Read the model definition and answer for the solid it produces. Units are mm, in the model's axes. A direction names the side the tool comes from. Round coordinates to 2 decimals unless told otherwise and drop trailing zeros. Write each loop counter-clockwise with the first axis right and the second up, starting at its lowest first coordinate (ties: lowest second). Pieces come first, ordered by that corner, then holes. Notation, with made-up numbers: (-33.75, 2) - (4.25, 2) arc R13 ccw to (4.25, 26) - close; hole circle Ø3 at (68.25, -30). An arc over 180 degrees is marked (long way). One line per item, written item: value. Start each with the question number.
(1) For faces 1 (the face through (36.164, 61.944, -12.114)), 2 (the face through (-30, 62, -5.797)), determine the directions among +Z, -Z, +X, -X, +Y, -Y from which every point of the face is accessible in a straight line to the end or side of a thin tool.
(2) A cutting plane is placed at B-B, the plane y = 21.5. Determine the outline of the cut face in (x, z), plus the area to 3 significant figures.
(3) A cutting plane is placed at C-C, the plane x = -8.5. Determine the outline of the cut face in (y, z).
(4) Find the intervals of material crossed by L1, parallel to Y at x = -16.5, z = -3.75; L2, parallel to X at y = 44.5, z = -0.5; L3, parallel to Z at x = -8.5, y = 5, in increasing order.
(5) The mould has two halves that part along Y. Classify faces 3 (the face through (-1.464, 4.056, -1.122)), 4 (the face through (15, 58, -6)), 5 (the face through (-13, 66, -4)): +Y half, -Y half, draft (parallel to the pull), parting line (faces both ways), or undercut.
(6) Flat-ended cylindrical pins translate along their axes: pin 1 Ø8 at (x, y) = (-16, 52.5) entering from +Z; pin 2 Ø2 at (y, z) = (53, -5) entering from -X; pin 3 Ø1.8 at (x, z) = (-35.79, -0.8) entering from +Y (1 decimal); pin 4 Ø2.5 at (x, y) = (-30, 63) entering from -Z. Find the tip coordinate at first contact, or state that the pin passes through.
(7) A cutting plane is placed at A-A, the plane x = -53. Determine the outline of the cut face in (y, z), plus the area to 3 significant figures.
from build123d import *

# Parameters (mm, degrees)
BOSS_EXTRUDE1_DEPTH = 8
SKETCH2_R           = 1.7
SKETCH2_R_2         = 1.5
CUT_EXTRUDE1_DEPTH  = 10
FILLET1_SIZE        = 5
SKETCH3_R           = 5
BOSS_EXTRUDE2_DEPTH = 25


with BuildPart() as part:
    # Sketch1 → Boss-Extrude1 (new body)
    with BuildSketch(Plane(origin=(0, 0, 0), x_dir=(1, 0, 0), z_dir=(0, 1, 0))):
        Polygon((0, 5.796570021), (-65, 5.796570021), (-65, -4.203429979), (0, -4.203429979), (42, 8.002969552), (39.5, 17.276398151), align=None)
    extrude(amount=BOSS_EXTRUDE1_DEPTH)

    # Sketch2 → Cut-Extrude1 (cut)
    with BuildSketch(Plane(origin=(0, 8, 0), x_dir=(1, 0, 0), z_dir=(0, 1, 0))):
        with Locations(Location((-59, 0.796570021, 0), (0, 0, 270))):
            Circle(SKETCH2_R)
        with Locations(Location((-53, 0.796570021, 0), (0, 0, 270))):
            Circle(SKETCH2_R_2)
        with Locations(Location((-35.792921067, 0.796570021, 0), (0, 0, 270))):
            Circle(SKETCH2_R_2)
        with Locations(Location((20.375, 6.319841926, 0), (0, 0, 270))):
            Circle(SKETCH2_R_2)
        with Locations(Location((35.015323176, 10.860923065, 0), (0, 0, 270))):
            Circle(SKETCH2_R)
        with Locations(Location((0, 0.796570021, 0), (0, 0, 270))):
            Circle(SKETCH2_R_2)
    extrude(amount=-CUT_EXTRUDE1_DEPTH, mode=Mode.SUBTRACT)

    # Fillet1
    # a fillet whose section is not a circle: 5 mm, written as the material it takes off along each edge
    with BuildSketch(Plane(origin=(-65, -12.5, 4.203429979), x_dir=(0, 0, -1), z_dir=(0, 1, 0)), Plane(origin=(-65, -12.5, -5.796570021), x_dir=(1, 0, 0), z_dir=(0, 1, 0))) as fillet1_piece_1:
        with BuildLine():
            Bezier((FILLET1_SIZE, 0), (0, 0), (0, -FILLET1_SIZE), weights=[1, 1, 1])
            Line((0, -FILLET1_SIZE), (0, 0))
            Line((0, 0), (FILLET1_SIZE, 0))
        make_face()
    extrude(amount=33, mode=Mode.SUBTRACT)

    # Fillet2
    # a fillet whose section is not a circle: 5 mm, written as the material it takes off along each edge
    with BuildSketch(Plane(origin=(39.5, -12.746283343, -17.276398151), x_dir=(-0.9602675163397548, 0, 0.27908116572545455), z_dir=(0, 1, 0))) as fillet2_piece_1:
        with BuildLine():
            Bezier((5.098513337, 0), (0, 0), (0.099464892, 5.097543034), weights=[1, 1, 1])
            Line((0.099464892, 5.097543034), (0, 0))
            Line((0, 0), (5.098513337, 0))
        make_face()
    extrude(amount=33.492566686, mode=Mode.SUBTRACT)
    with BuildSketch(Plane(origin=(42, -12.258475337, -8.002969552), x_dir=(-0.2602945720874772, 0, -0.9655292516241013), z_dir=(0, 1, 0))) as fillet2_piece_2:
        with BuildLine():
            Bezier((4.903390135, 0), (0, 0), (-0.09565831, 4.902456966), weights=[1, 1, 1])
            Line((-0.09565831, 4.902456966), (0, 0))
            Line((0, 0), (4.903390135, 0))
        make_face()
    extrude(amount=32.516950674, mode=Mode.SUBTRACT)

    # Sketch3 → Boss-Extrude2 (add)
    with BuildSketch(Plane(origin=(0, 8, 0), x_dir=(1, 0, 0), z_dir=(0, 1, 0))):
        with Locations(Location((-10.792921067, 0.796570021, 0), (0, 0, 270))):
            Circle(SKETCH3_R)
    extrude(amount=BOSS_EXTRUDE2_DEPTH)

    # Mirror3: part across plane


with BuildPart() as part_1:
    add(part.part)
    add(part.part.mirror(Plane.ZX.offset(33)))


solid = part_1.part
Here are the results:
1. face 1: +Y, -Y
1. face 2: -Z, -X, +Y, -Y
2. outline: circle Ø10 at (-10.79, -0.8)
2. area: 78.5 mm²
3. outline: (0, -5.8) - (8, -5.8) - (8, -5.24) - (58, -5.24) - (58, -5.8) - (66, -5.8) - (66, 4.2) - (58, 4.2) - (58, 3.65) - (8, 3.65) - (8, 4.2) - (0, 4.2) - close
4. L1: 0 to 8, 58 to 66
4. L2: -15.78 to -5.8
4. L3: -5.8 to 4.2
5. face 3: draft
5. face 4: undercut
5. face 5: +Y half
6. pin 1: z = 4.06
6. pin 2: x = -14.63
6. pin 3: through
6. pin 4: z = -5.8
7. outline: (0, -5.8) - (8, -5.8) - (8, -2.3) - (0, -2.3) - close; (0, 0.7) - (8, 0.7) - (8, 4.2) - (0, 4.2) - close; (58, -5.8) - (66, -5.8) - (66, -2.3) - (58, -2.3) - close; (58, 0.7) - (66, 0.7) - (66, 4.2) - (58, 4.2) - close
7. area: 112 mm²
